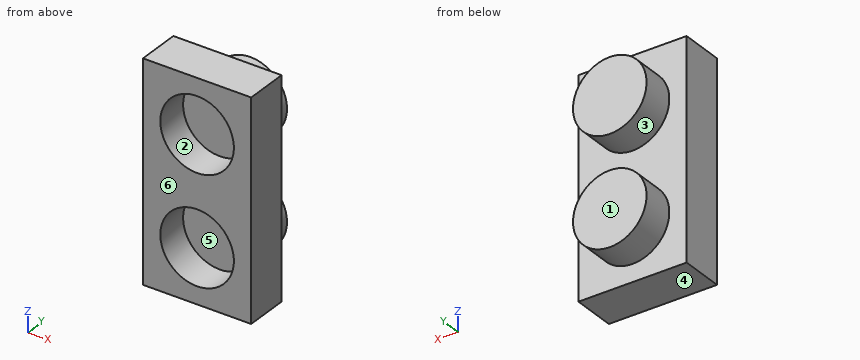
Autodesk Inventor part; units mm, degrees
ref_plane "YZ Plane" through (0, 0, 0) normal (1, 0, 0) x (0, 1, 0)
ref_plane "XZ Plane" through (0, 0, 0) normal (0, 1, 0) x (-1, 0, 0)
ref_plane "XY Plane" through (0, 0, 0) normal (0, 0, 1) x (1, 0, 0)
sketch "草圖1" plane through (0, 0, 0) normal (0, 1, 0) x (-1, 0, 0)
  line L0 (2.5, 5) -> (-2.5, 5)
  line L1 (-2.5, 5) -> (-2.5, -5)
  line L2 (-2.5, -5) -> (2.5, -5)
  line L3 (2.5, -5) -> (2.5, 5)
  circle A0 centre (0, 2.5) radius 1.7
  line L4 (2.5, 0) -> (-2.5, 0) construction
  circle A1 centre (0, -2.5) radius 1.7
  point P0 (0, 0)
  point P1 (0, -5)
  point P2 (0, 5)
  dimension "d0" = 5
  dimension "d1" = 10
  dimension "d2" = 3.4
  dimension "d3" = 2.5
extrude "擠出1" add sketch "草圖1" along normal blind 2 contours L3 L2 L1 L0 | A0 | A1
extrude "擠出2" cut sketch "草圖1" along normal blind 1.5 contours A0 | A1
sketch "草圖2" plane through (0, 2, 0) normal (0, 1, 0) x (1, 0, 0)
  circle A0 centre (0, -2.5) radius 1.7
  circle A1 centre (0, 2.5) radius 1.7
  point P0 (0, 0)
extrude "擠出3" add sketch "草圖2" along normal blind 1.5
properties part number "110033226_ipt_13_草地二"
Geometry: final body of the model. Coordinates: model frame, mm. Face numbers are marked on the shaded views. A direction names the side the tool comes from. Coordinates: 2 decimals unless noted, no trailing zeros. Order: outer loops, then holes, each group sorted by start corner. A loop starts at its lowest first (then second) coordinate and runs counter-clockwise, first axis right, second up. Notation, with made-up numbers: (39, 40.5) -> (46, 40.5) arc R25 cw to (46, 77.5) -> close; hole circle Ø7 at (40, 25.5). An arc over 180 degrees is marked (long way). Answer in a Markdown table with one row per item.
Item 1: Section C-C on z = -3. Output: boundary loops of the cut face in (x, y).
Return value:
| item | result |
|---|---|
| outline | (-2.5, 0) -> (-1.62, 0) -> (-1.62, 1.5) -> (1.62, 1.5) -> (1.62, 0) -> (2.5, 0) -> (2.5, 2) -> (1.62, 2) -> (1.62, 3.5) -> (-1.62, 3.5) -> (-1.62, 2) -> (-2.5, 2) -> close |
Item 2: Section A-A on y = 0.95. Output: boundary loops of the cut face in (x, z).
Return value:
| item | result |
|---|---|
| outline | (-2.5, -5) -> (2.5, -5) -> (2.5, 5) -> (-2.5, 5) -> close; hole circle Ø3.4 at (0, -2.5); hole circle Ø3.4 at (0, 2.5) |
Item 3: Draft query along Z for the marked faces 4, 5 and 6. Return one class per face: released by +Z, released by -Z, zero draft, split by the parting line, or undercut.
Return value:
| item | result |
|---|---|
| face 4 | released by -Z |
| face 5 | undercut |
| face 6 | zero draft |
Item 4: Access query for the marked faces 1, 2 and 3. Directions: +Z, -Z, +X, -X, +Y, -Y. A direction counts if a zero-diameter tool reaches every point of the face in a straight line with its end or side. Return the directions, or none.
Return value:
| item | result |
|---|---|
| face 1 | +Z, -Z, +X, -X, +Y |
| face 2 | -Y |
| face 3 | +Y |
Item 5: Section B-B on y = 3. Output: boundary loops of the cut face in (x, z), plus the area to 3 significant figures.
Return value:
| item | result |
|---|---|
| outline | circle Ø3.4 at (0, -2.5); circle Ø3.4 at (0, 2.5) |
| area | 18.2 mm² |
Item 6: Contact query for flat-ended pins moving along their axis: P1, Ø1.7, axis at x = 0.5, z = -2.5, coming from the -Y side; P2, Ø1.5, axis at x = -1, y = 2.5, coming from the +Z side; P3, Ø1.5, axis at y = 3, z = 3.5, coming from the -X side. Output: stop coordinate, or through.
Return value:
| item | result |
|---|---|
| P1 | stops at y = 1.5 |
| P2 | stops at z = 5 |
| P3 | stops at x = -1.68 |
Item 7: Ray query, L1, parallel to Z at x = 0, y = 0.8; L2, parallel to Z at x = -0.9, y = 1.1; L3, parallel to Y at x = 2.05, z = -3.5. Return the intervals inside material, ascending.
Return value:
| item | result |
|---|---|
| L1 | z = -5 to -4.2, -0.8 to 0.8, 4.2 to 5 |
| L2 | z = -5 to -3.94, -1.06 to 1.06, 3.94 to 5 |
| L3 | y = 0 to 2 |
Item 8: Section D-D on x = 0.75. Output: boundary loops of the cut face in (y, z).
Return value:
| item | result |
|---|---|
| outline | (0, -5) -> (2, -5) -> (2, -4.03) -> (3.5, -4.03) -> (3.5, -0.97) -> (2, -0.97) -> (2, 0.97) -> (3.5, 0.97) -> (3.5, 4.03) -> (2, 4.03) -> (2, 5) -> (0, 5) -> (0, 4.03) -> (1.5, 4.03) -> (1.5, 0.97) -> (0, 0.97) -> (0, -0.97) -> (1.5, -0.97) -> (1.5, -4.03) -> (0, -4.03) -> close |
